CAD build for the part. Positions are in the model's coordinates, mm. Coordinates: 2 decimals unless noted, no trailing zeros. Write each loop counter-clockwise with the first axis right and the second up, starting at its lowest first coordinate (ties: lowest second). Pieces come first, ordered by that corner, then holes. Notation, with made-up numbers: (58.5, 21.5) -> (98.5, 21.5) arc R20 ccw to (98.5, 41.5) -> close; hole circle Ø2 at (21.5, -5.5). An arc over 180 degrees is marked (long way). Answer as CSV lines item,"result". Start each with the question number.
```python
from build123d import *

# Parameters (mm, degrees)
SALIENTE_EXTRUIR1_DEPTH = 50
CROQUIS2_W              = 50
CROQUIS2_H              = 50
SALIENTE_EXTRUIR2_DEPTH = 150
SALIENTE_EXTRUIR3_DEPTH = 50


with BuildPart() as part:
    # Croquis1 → Saliente-Extruir1 (new body)
    with BuildSketch(Plane(origin=(0, 0, 0), x_dir=(0, 0, -1), z_dir=(1, 0, 0))):
        Polygon((0, 0), (0, 600), (-1800, 600), (-1800, 0), (-1750, 0), (-1750, 550), (-50, 550), (-50, 0), align=None)
    extrude(amount=SALIENTE_EXTRUIR1_DEPTH)

    # Croquis2 → Saliente-Extruir2 (add)
    with BuildSketch(Plane.ZY):
        with Locations((1775, 300)):
            Rectangle(CROQUIS2_W, CROQUIS2_H)
        with Locations((25, 300)):
            Rectangle(CROQUIS2_W, CROQUIS2_H)
    extrude(amount=SALIENTE_EXTRUIR2_DEPTH)

    # Croquis3 → Saliente-Extruir3 (add)
    with BuildSketch(Plane.ZY.offset(150)):
        Polygon((1750, 0), (1800, 0), (1800, 600), (0, 600), (0, 0), (50, 0), (50, 550), (1750, 550), align=None)
    extrude(amount=SALIENTE_EXTRUIR3_DEPTH)


solid = part.part
```
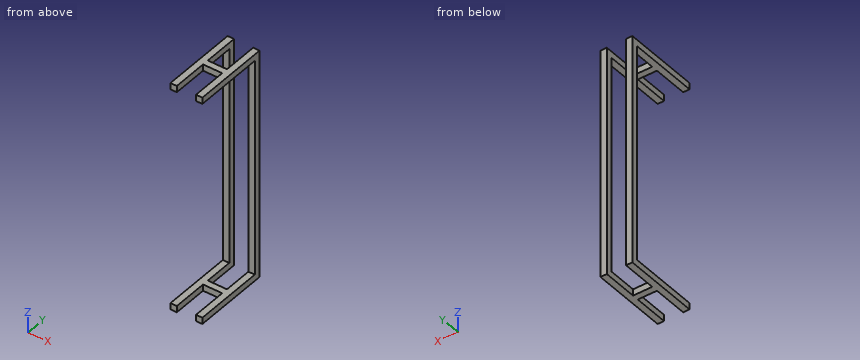
1. Cut at A-A (y = 506.5). Give the cut face in (x, z), then the cut area to 3 significant figures.
2. Cut at C-C (z = 215). Give the cut face in (x, y).
3. Cut at B-B (x = -68.5). Give the cut face in (y, z).
4. Cut at D-D (x = 17). Give the cut face in (y, z).
5. Flat gauge pins, fed straight in: P1, Ø15, axis at x = -186, z = 1170.5, coming from the -Y side; P2, Ø15, axis at x = -81, z = 15.5, coming from the +Y side. Where does each tip first touch, or does it go through?
6. Wall check: line 1 (Z direction, x = -161.5, y = 113); line 2 (Y direction, x = 27.5, z = 390). Give the ranges that are in metal, low to high.
Geometry check:
1,outline,"(-200, 0) -> (-150, 0) -> (-150, 50) -> (-200, 50) -> close; (-200, 1750) -> (-150, 1750) -> (-150, 1800) -> (-200, 1800) -> close; (0, 0) -> (50, 0) -> (50, 50) -> (0, 50) -> close; (0, 1750) -> (50, 1750) -> (50, 1800) -> (0, 1800) -> close"
1,area,"10,000 mm²"
2,outline,"(-200, 550) -> (-150, 550) -> (-150, 600) -> (-200, 600) -> close; (0, 550) -> (50, 550) -> (50, 600) -> (0, 600) -> close"
3,outline,"(275, 0) -> (325, 0) -> (325, 50) -> (275, 50) -> close; (275, 1750) -> (325, 1750) -> (325, 1800) -> (275, 1800) -> close"
4,outline,"(0, 0) -> (600, 0) -> (600, 1800) -> (0, 1800) -> (0, 1750) -> (550, 1750) -> (550, 50) -> (0, 50) -> close"
5,P1,"y = 550"
5,P2,"y = 325"
6,line 1,"0 to 50, 1750 to 1800"
6,line 2,"550 to 600"
